For this review, take the finished solid that the model builds, in its own axes (mm). A direction names the side the tool comes from. Coordinates: 2 decimals unless noted, no trailing zeros. Write each loop counter-clockwise with the first axis right and the second up, starting at its lowest first coordinate (ties: lowest second). Pieces come first, ordered by that corner, then holes. Notation, with made-up numbers: (34, 1) -> (93, 1) arc R21 ccw to (93, 18) -> close; hole circle Ø10 at (2, 84.25). An arc over 180 degrees is marked (long way). One line per item, written item: value. Start each with the question number.
1) For probe 1 along Y at (x, z) = (-11.25, 19); probe 2 along Y at (x, z) = (-3.25, 73); probe 3 along X at (y, z) = (-27.25, 169), list the stretches that pass through material, from the lowest coordinate up. Write a range as from..to.
2) Add section C-C (z = 30.5). State the section outline as (x, y) points.
3) Machinability: for faces 5 (the flat face through (-6.713, -27, 89)), 6 (the cylindrical face through (0, -21, 89)), which of the approach directions +Z, -Z, +X, -X, +Y, -Y give a long, thin tool a straight path to every point of the face, cutting with its end or side? Answer none if there is none.
4) For pin 1 Ø8 at (x, z) = (-3, 133.5) entering from -Y; pin 2 Ø5 at (y, z) = (-32, 124) entering from -X; pin 3 Ø6.5 at (y, z) = (-26.5, 112) entering from +X; pin 4 Ø1.5 at (x, y) = (0.5, -19.5) entering from +Z, all flat-tipped, find the tip position at first contact; note any pin that passes through.
5) Add section A-A (y = -27). State the section outline as (x, z) points, and give its area (3 significant figures).
6) Mouldability with a two-part tool opening along X and no side actions: class faces 1 (the flat face through (0, -22, 0)), 2 (the flat face through (-13.304, -22.59, 88.74)), 3 (the flat face through (4.287, -27, 89)), 4 (the flat face through (-2.966, -31.936, 88.74)) as released by +X, released by -X, zero draft, split by the parting line, or undercut.
7) Add section D-D (x = 8.5). State the section outline as (y, z) points, and give its area (3 significant figures).
8) Add section B-B (x = -3.5). State the section outline as (y, z) points.
from build123d import *

# Parameters (mm, degrees)
F1_DEPTH    = 180
F2_R        = 5
F3_T1_DEPTH = 189.5214724234


# Not quite as in the source:
# - a fillet or chamfer that OpenCascade refuses, or shapes differently, is made with other operations: its cross-section is extruded or revolved along the edge and cut away or added


with BuildPart() as f1:
    # F0 (on Top) → F1 (new body)
    with BuildSketch(Plane.XY):
        with BuildLine():
            ThreePointArc((14.1226732436, -15.5418821401), (0.1645874713, -20.9993550131), (-13.8773267564, -15.7613388421))
            Line((-13.8773267564, -15.7613388421), (-12.7134246975, -29.6120676683))
            Line((-12.7134246975, -29.6120676683), (-6.7134246975, -29.6071426253))
            Line((-6.7134246975, -29.6071426253), (-6.7134246975, -23.6071426253))
            Line((-6.7134246975, -23.6071426253), (4.2865298223, -23.6563930556))
            Line((4.2865298223, -23.6563930556), (4.2865298223, -29.6071426253))
            Line((4.2865298223, -29.6071426253), (6.2865237583, -29.6120676683))
            Line((6.2865237583, -29.6120676683), (6.2766736722, -33.6120555403))
            Line((6.2766736722, -33.6120555403), (-12.4721404439, -30.2120676683))
            Line((-12.4721404439, -30.2120676683), (-12.4721404439, -31.7862083661))
            ThreePointArc((-12.4721404439, -31.7862083661), (-1.3967093827, -36.1708063262), (10.2766736722, -38.5418821401))
            Line((10.2766736722, -38.5418821401), (14.1226732436, -15.5418821401))
        make_face()
    extrude(amount=F1_DEPTH)

    # F2
    f2_edges = [f1.edges().sort_by_distance(p)[0] for p in [
        (10.276674, -38.541882, 90),
    ]]
    fillet(f2_edges, radius=F2_R)

    # F3: fillet of radius 3 on 1 edges, made by hand

    # F3_s2 → F3_t1 (cut)
    with BuildSketch(Plane.XY.offset(-4.7607362117)):
        with BuildLine():
            ThreePointArc((-10.7583691092, -32.6164645294), (-11.9315343306, -31.6396992801), (-12.4721404439, -30.2120676683))
            Line((-12.4721404439, -30.2120676683), (-12.4721404439, -31.7862083661))
            ThreePointArc((-12.4721404439, -31.7862083661), (-11.618180513, -32.2073755998), (-10.7583691092, -32.6164645294))
        make_face()
    extrude(amount=F3_T1_DEPTH, mode=Mode.SUBTRACT)


solid = f1.part
Numbers:
1. probe 1: -32.33..-30.43, -29.61..-17.73
1. probe 2: -35.59..-31.88, -23.62..-20.75
1. probe 3: -12.91..-6.71, 4.29..12.16
2. outline: (-13.88, -15.76) -> (-12.71, -29.61) -> (-6.71, -29.61) -> (-6.71, -23.61) -> (4.29, -23.66) -> (4.29, -29.61) -> (6.29, -29.61) -> (6.28, -33.61) -> (-12.47, -30.21) arc R3 ccw to (-10.76, -32.62) arc R67.55 ccw to (5.22, -37.78) arc R5 ccw to (11.09, -33.69) -> (14.12, -15.54) arc R21 cw to start
3. face 5: +Z, -Z
3. face 6: +Z, -Z, +Y
4. pin 1: y = -36.83
4. pin 2: x = -12.72
4. pin 3: x = 12.83
4. pin 4: through
5. outline: (-12.93, 0) -> (-6.71, 0) -> (-6.71, 180) -> (-12.93, 180) -> close; (4.29, 0) -> (12.21, 0) -> (12.21, 180) -> (4.29, 180) -> close
5. area: 2,550 mm²
6. face 1: zero draft
6. face 2: released by -X
6. face 3: undercut
6. face 4: undercut
7. outline: (-37.28, 0) -> (-19.2, 0) -> (-19.2, 180) -> (-37.28, 180) -> close
7. area: 3,250 mm²
8. outline: (-35.51, 0) -> (-31.84, 0) -> (-31.84, 180) -> (-35.51, 180) -> close; (-23.62, 0) -> (-20.71, 0) -> (-20.71, 180) -> (-23.62, 180) -> close
